Geometry check sheet. Reference: the model listing, model coordinates, mm. A direction names the side the tool comes from. Coordinates: 2 decimals unless noted, no trailing zeros. Loops run counter-clockwise (first coordinate to the right, second up) from the corner with the lowest first, then second, coordinate; pieces in that order, holes last. Notation, with made-up numbers: (53.5, 0.25) - (65.5, 0.25) arc R23 cw to (65.5, 16.25) - close; hole circle Ø2 at (24, 82.5). An arc over 180 degrees is marked (long way). One line per item, written item: value.
from build123d import *

# Parameters (mm, degrees)
F0_W          = 101.6
F0_H          = 127
F0_W_2        = 88.9
F0_H_2        = 114.3
F1_DEPTH      = 1524
F1_DEPTH_BACK = 25.4
F2_R          = 16.764
F3_DEPTH      = 127


# Not quite as in the source:
# - a feature names something its author has since deleted; it is built from what else it names


with BuildPart() as f1:
    # F0 (on Front) → F1 (new body, two sides)
    with BuildSketch(Plane.XZ) as f1_sk:
        with Locations((-14.2066246522, 5.0925366492)):
            Rectangle(F0_W, F0_H)
        with Locations((-14.2066246522, 5.0925366492)):
            Rectangle(F0_W_2, F0_H_2, mode=Mode.SUBTRACT)
    extrude(amount=F1_DEPTH)
    extrude(f1_sk.sketch, amount=-F1_DEPTH_BACK)

    # F2 (on face) → F3 (cut)
    with BuildSketch(Plane.YZ.offset(36.5933753478)):
        with Locations((-1405.636, 21.8565366492)):
            Circle(F2_R)
    extrude(amount=-F3_DEPTH, mode=Mode.SUBTRACT)


solid = f1.part
(1) Cross-section at C-C on y = -291.5. Record the cut outline in (x, z), and give its area (3 significant figures).
Reply:
outline: (-65.01, -58.41) - (36.59, -58.41) - (36.59, 68.59) - (-65.01, 68.59) - close; hole (-58.66, -52.06) - (30.24, -52.06) - (30.24, 62.24) - (-58.66, 62.24) - close
area: 2,740 mm2
(2) Release check for a two-part mould opening along X. For faces 1 (the face through (33.46, -1418.94, 11.66)), 2 (the face through (-15, -760, -52.057)), 3 (the face through (-65.007, -760, 4)) record: pulls with the +X half, pulls with the -X half, needs draft (parallel to the pull), parting line crosses it, or undercut.
Reply:
face 1: needs draft
face 2: undercut
face 3: pulls with the -X half
(3) Cross-section at A-A on z = -32. Record the cut outline in (x, y).
Reply:
outline: (-65.01, -1524) - (-58.66, -1524) - (-58.66, 25.4) - (-65.01, 25.4) - close; (30.24, -1524) - (36.59, -1524) - (36.59, 25.4) - (30.24, 25.4) - close
(4) Access from +Z, -Z, +X, -X, +Y, -Y to the whole of each face (thin tool, end or side, straight path). Record for faces 4 (the face through (36.593, -760, 4)), 5 (the face through (-15, -760, 62.243)).
Reply:
face 4: +Z, -Z, +X, +Y, -Y
face 5: +Y, -Y
(5) Cross-section at B-B on x = -46. Record the cut outline in (y, z).
Reply:
outline: (-1524, -58.41) - (25.4, -58.41) - (25.4, -52.06) - (-1524, -52.06) - close; (-1524, 62.24) - (25.4, 62.24) - (25.4, 68.59) - (-1524, 68.59) - close
(6) Material ranges on probe 1 along Z at (x, y) = (25, -632); probe 2 along X at (y, z) = (-1346.5, -11), recorded low to high. Write a range as from..to.
Reply:
probe 1: -58.41..-52.06, 62.24..68.59
probe 2: -65.01..-58.66, 30.24..36.59
